from build123d import *

# Parameters (mm, degrees)
F0_W      = 40
F0_H      = 30
F1_DEPTH  = 10
F2_R      = 5
F3_T      = -3
F4_W      = 28
F4_H      = 3
F5_DEPTH  = 3
F6_W      = 32.3581136763
F6_H      = 60.2468792349
F7_DEPTH  = 25
F8_R      = 0.75
F9_DEPTH  = 0.75
F10_R     = 0.74999
F11_W     = 14
F11_H     = 3
F12_DEPTH = 0.2
F13_R     = 1
F15_W     = 15
F15_H     = 2.3
F16_DEPTH = 3


# Not quite as in the source:
# - a fillet or chamfer is up to 0.001 mm smaller than in the source, because OpenCascade refuses the exact size


with BuildPart() as f1:
    # F0 (on Top) → F1 (new body)
    with BuildSketch(Plane.XY):
        Rectangle(F0_W, F0_H)
    extrude(amount=-F1_DEPTH)

    # F2
    f2_edges = [f1.edges().sort_by_distance(p)[0] for p in [
        (20, 0, -10),
        (0, 15, -10),
        (-20, 0, -10),
        (0, -15, -10),
    ]]
    fillet(f2_edges, radius=F2_R)

    # F3
    f3_openings = [f1.faces().sort_by_distance(p)[0] for p in [
        (0, 0, 0),
    ]]
    offset(amount=F3_T, openings=f3_openings)

    # F4 (on face) → F5 (cut)
    with BuildSketch(Plane.XY):
        with Locations((0, 13.5)):
            Rectangle(F4_W, F4_H)
    extrude(amount=-F5_DEPTH, mode=Mode.SUBTRACT)

    # F6 (on Top) → F7 (cut)
    with BuildSketch(Plane.XY):
        with Locations((16.1790568382, -2.0559011027)):
            Rectangle(F6_W, F6_H)
    extrude(amount=-F7_DEPTH, mode=Mode.SUBTRACT)

    # F8 (on face) → F9 (cut)
    with BuildSketch(Plane.YZ.offset(-14)):
        with Locations((13.5, -1.5)):
            Circle(F8_R)
    extrude(amount=-F9_DEPTH, mode=Mode.SUBTRACT)

    # F10 (radius 0.75 in the source; OpenCascade refuses exactly that, so slightly less here)
    f10_edges = [f1.edges().sort_by_distance(p)[0] for p in [
        (-14.75, 12.75, -1.5),
    ]]
    fillet(f10_edges, radius=F10_R)

    # F11 (on face) → F12 (cut)
    with BuildSketch(Plane.XY.offset(-3)):
        with Locations((-7, 13.5)):
            Rectangle(F11_W, F11_H)
    extrude(amount=-F12_DEPTH, mode=Mode.SUBTRACT)

    # F13
    f13_edges = [f1.edges().sort_by_distance(p)[0] for p in [
        (-17, 15, 0),
        (-15.5, 12, 0),
        (-7, 15, -3.2),
        (-7, 12, -3.2),
    ]]
    fillet(f13_edges, radius=F13_R)

    # F14: F1 across plane


with BuildPart() as f1_1:
    add(f1.part)
    add(f1.part.mirror(Plane.YZ))

    # F15 (on face) → F16 (cut, through all)
    with BuildSketch(Plane.XZ.offset(15)):
        with Locations((0, -3.15)):
            Rectangle(F15_W, F15_H)
    extrude(amount=-F16_DEPTH, mode=Mode.SUBTRACT)


solid = f1_1.part
Geometry check sheet. Reference: the model listing, model coordinates, mm. A direction names the side the tool comes from. Give positions to 0.01 mm unless a question says otherwise; leave off trailing zeros. Loops run counter-clockwise (first coordinate to the right, second up) from the corner with the lowest first, then second, coordinate; pieces in that order, holes last. Notation, with made-up numbers: M -11,-31 L 32,-31 A26 ccw 32,-7 Z; hole C 3,82.5 d3. An arc over 180 degrees is marked long. Answer as a JSON object with one key per item and string values. Group by question number.
Item 1: Access from +Z, -Z, +X, -X, +Y, -Y to the whole of each face (thin tool, end or side, straight path). Record for faces 1 (the flat face through (0.3, 15, -4.7)), 2 (the flat face through (0, -14, -4.3)), 3 (the cylindrical face through (-0.196, 12.301, -3.485)).
Item 2: Material ranges on L1, parallel to Y at x = 14.05, z = -1.5; L2, parallel to X at y = -3, z = -1.75; L3, parallel to Y at x = -12.5, z = -5, recorded low to high.
Item 3: Gauge pin test, flat ends, axial feed: pin 1 (2 mm diameter, centred on x = 9, z = -9, fed in from +Y); pin 2 (3.5 mm diameter, centred on x = 0, y = -14, fed in from -Z); pin 3 (16 mm diameter, centred on x = 7.5, y = 3.5, fed in from +Z). Record the tip position at first contact, or that the pin passes through.
Item 4: Sectioned sample at D-D on y = -4.5. Record the boundary of the cut face in (x, z).
Item 5: Mould release check, pull along Z, two halves, no side actions. Record for faces 4 (the cylindrical face through (-16.958, 14.699, -0.285)), 5 (the cylindrical face through (19, 0, -8)), 6 (the flat face through (0, -14, -2)): pulls with the +Z half, pulls with the -Z half, needs draft (parallel to the pull), parting line crosses it, or undercut.
Item 6: Sectioned sample at C-C on z = -5.5. Record the boundary of the cut face in (x, y), plus the area to 3 significant figures.
Item 7: Sectioned sample at A-A on x = -2. Record the boundary of the cut face in (y, z), plus the area to 3 significant figures.
Item 8: Sectioned sample at B-B on x = 13. Record the boundary of the cut face in (y, z).
Findings below:
{
 "1": {"face 1": "+Z, -Z, +X, -X, +Y", "face 2": "-Y", "face 3": "+Z"},
 "2": {"L1": "-15 to -12, 12 to 12.75, 14.25 to 15", "L2": "-20 to -17, 17 to 20", "L3": "-15 to -12, 12 to 15"},
 "3": {"pin 1": "y = 14", "pin 2": "z = -9.47", "pin 3": "z = -6.32"},
 "4": {"outline": "M -20,-5 A5 ccw -15,-10 L 15,-10 A5 ccw 20,-5 L 20,0 L 17,0 L 17,-5 A2 cw 15,-7 L -15,-7 A2 cw -17,-5 L -17,0 L -20,0 Z"},
 "5": {"face 4": "pulls with the +Z half", "face 5": "pulls with the -Z half", "face 6": "undercut"},
 "6": {"outline": "M -19.97,-14.97 L 19.97,-14.97 L 19.97,14.97 L -19.97,14.97 Z; hole M -16.94,-11.94 L 16.94,-11.94 L 16.94,11.94 L -16.94,11.94 Z", "area": "388 mm2"},
 "7": {"outline": "M -15,-5 A5 ccw -10,-10 L 10,-10 A5 ccw 15,-5 L 15,-4.2 A1 ccw 14,-3.2 L 13,-3.2 A1 ccw 12,-4.2 L 12,-5 A2 cw 10,-7 L -10,-7 A2 cw -12,-5 L -12,-4.3 L -15,-4.3 Z; M -15,-2 L -12,-2 L -12,0 L -15,0 Z", "area": "106 mm2"},
 "8": {"outline": "M -15,-5 A5 ccw -10,-10 L 10,-10 A5 ccw 15,-5 L 15,-4.2 A1 ccw 14,-3.2 L 13,-3.2 A1 ccw 12,-4.2 L 12,-5 A2 cw 10,-7 L -10,-7 A2 cw -12,-5 L -12,0 L -15,0 Z"}
}
